Model file for the job. Use its own axes, mm. Coordinates: 2 decimals unless noted, no trailing zeros. Write each loop counter-clockwise with the first axis right and the second up, starting at its lowest first coordinate (ties: lowest second). Pieces come first, ordered by that corner, then holes.
Q1. Band-saw the part on B-B, the plane x = -10.75. Write the cut outline in (y, z).
Q2. Band-saw the part on A-A, the plane z = 126. Write the cut outline in (x, y).
Q3. Band-saw the part on C-C, the plane x = -29.25. Write the cut outline in (y, z).
Q4. Drill centre lines: probe 1 along X at (y, z) = (1.4, -126); probe 2 along Z at (x, y) = (-46.75, 3.85); probe 3 along Z at (x, y) = (28.25, 1.45). Where is each one in solid material? Low to high.
Q5. Pin check, flat tip, straight feed: P1, Ø4.5, axis at x = 10.75, z = 126, coming from the -Y side. Stop position of the tip, or through.
from build123d import *

# Parameters (mm, degrees)
SKIZZE1_W                       = 72.5
SKIZZE1_H                       = 268
AUFSATZ_LINEAR_AUSTRAGEN1_DEPTH = 5
M6_GEWINDEBOHRUNG2_D            = 5
M6_GEWINDEBOHRUNG2_DEPTH        = 5
M6_GEWINDEBOHRUNG1_D            = 5
M6_GEWINDEBOHRUNG1_DEPTH        = 5
SKIZZE7_W                       = 268
SKIZZE7_H                       = 5
AUFSATZ_LINEAR_AUSTRAGEN2_DEPTH = 18.5
M6_GEWINDEBOHRUNG3_D            = 5
M6_GEWINDEBOHRUNG3_DEPTH        = 5


with BuildPart() as part:
    # Skizze1 → Aufsatz-Linear austragen1 (new body)
    with BuildSketch(Plane(origin=(0, 0, 0), x_dir=(1, 0, 0), z_dir=(0, 1, 0))):
        Rectangle(SKIZZE1_W, SKIZZE1_H)
    extrude(amount=AUFSATZ_LINEAR_AUSTRAGEN1_DEPTH)

    # M6 Gewindebohrung2
    with Locations(Plane(origin=(0, 5, 0), x_dir=(1, 0, 0), z_dir=(0, 1, 0))):
        with Locations((-29.25, -126), (10.75, -126), (-29.25, 126), (10.75, 126)):
            Hole(M6_GEWINDEBOHRUNG2_D / 2, depth=M6_GEWINDEBOHRUNG2_DEPTH)

    # M6 Gewindebohrung1
    with Locations(Plane(origin=(0, 5, 0), x_dir=(1, 0, 0), z_dir=(0, 1, 0))):
        with Locations((29.25, 30.2), (-10.75, 30.2)):
            Hole(M6_GEWINDEBOHRUNG1_D / 2, depth=M6_GEWINDEBOHRUNG1_DEPTH)

    # Skizze7 → Aufsatz-Linear austragen2 (add)
    with BuildSketch(Plane.ZY.offset(36.25)):
        with Locations((0, 2.5)):
            Rectangle(SKIZZE7_W, SKIZZE7_H)
    extrude(amount=AUFSATZ_LINEAR_AUSTRAGEN2_DEPTH)

    # M6 Gewindebohrung3
    with Locations(Plane(origin=(0, 5, 0), x_dir=(1, 0, 0), z_dir=(0, 1, 0))):
        with Locations((-46.75, -126), (28.25, -126), (28.25, 126), (-46.75, 126)):
            Hole(M6_GEWINDEBOHRUNG3_D / 2, depth=M6_GEWINDEBOHRUNG3_DEPTH)


solid = part.part
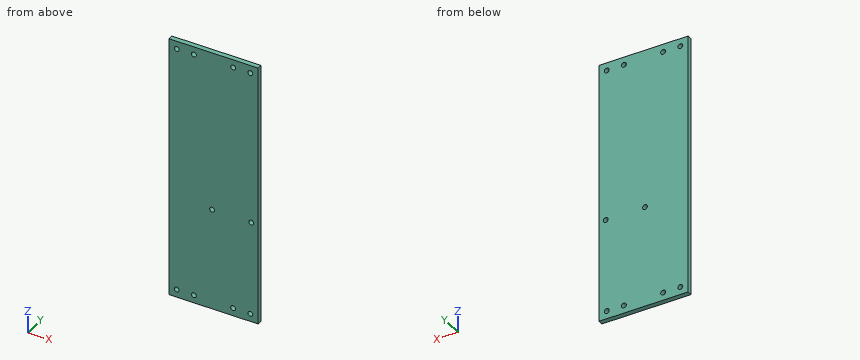
Answer sheet:
1. outline: (0, -134) - (5, -134) - (5, -32.7) - (0, -32.7) - close; (0, -27.7) - (5, -27.7) - (5, 134) - (0, 134) - close
2. outline: (-54.75, 0) - (-49.25, 0) - (-49.25, 5) - (-54.75, 5) - close; (-44.25, 0) - (-31.75, 0) - (-31.75, 5) - (-44.25, 5) - close; (-26.75, 0) - (8.25, 0) - (8.25, 5) - (-26.75, 5) - close; (13.25, 0) - (25.75, 0) - (25.75, 5) - (13.25, 5) - close; (30.75, 0) - (36.25, 0) - (36.25, 5) - (30.75, 5) - close
3. outline: (0, -134) - (5, -134) - (5, -128.5) - (0, -128.5) - close; (0, -123.5) - (5, -123.5) - (5, 123.5) - (0, 123.5) - close; (0, 128.5) - (5, 128.5) - (5, 134) - (0, 134) - close
4. probe 1: x = -54.75 to -49.25, -44.25 to -31.75, -26.75 to 8.25, 13.25 to 25.75, 30.75 to 36.25
4. probe 2: z = -134 to -128.5, -123.5 to 123.5, 128.5 to 134
4. probe 3: z = -134 to -128.5, -123.5 to -32.49, -27.91 to 123.5, 128.5 to 134
5. P1: passes through
